Design review of the part built by this model. Coordinates are the model's own, in mm. A direction names the side the tool comes from. Coordinates: 2 decimals unless noted, no trailing zeros. Loops run counter-clockwise (first coordinate to the right, second up) from the corner with the lowest first, then second, coordinate; pieces in that order, holes last. Notation, with made-up numbers: M -30,48.5 L 9,48.5 A25 cw 9,79.5 Z; hole C -12,13.5 d5. An arc over 180 degrees is marked long. Put each result on its own line as item: value. Start each with the question number.
(1) Take a section at D-D, the plane z = -21. Give the boundary of the cut face in (x, y).
(2) Take a section at C-C, the plane x = -104. Give the boundary of the cut face in (y, z), then the cut area to 3 significant figures.
(3) Take a section at A-A, the plane y = 34.5. Give the boundary of the cut face in (x, z), then the cut area to 3 significant figures.
(4) Clearance check with flat-ended pins moving along their axes: pin 1 (4.5 mm diameter, centred on x = -11, z = 28.35, fed in from +Y); pin 2 (5.5 mm diameter, centred on y = 54.15, z = -25.11, fed in from +X); pin 3 (5 mm diameter, centred on x = -126, y = 72.5, fed in from -Z); pin 4 (2 mm diameter, centred on x = -129, z = -28.35, fed in from +Y). State where each tip first meets the part, or that it passes through.
(5) Take a section at B-B, the plane y = 66.5. Give the boundary of the cut face in (x, z).
(6) For faces 1 (the cylindrical face through (-17.787, 53.146, 26.424)), 2 (the flat face through (-69, 15, 0)), 3 (the flat face through (2, 2, 0)), 4 (the flat face through (-69, 17, 0)), list the 3-axis set-ups (+Z, -Z, +X, -X, +Y, -Y) from which the entire face can be reached by the end or side of a thin tool; tool diameter is ignored.
(7) The part is to be moulded in two halves that separate along Z. For faces 5 (the flat face through (-70, 16, -33.35)), 6 (the cylindrical face through (-10, 0.82, -29.66)), 7 (the flat face through (-20, 7, 0)), say which applies: +Z half, -Z half, draft (parallel to the pull), parting line (faces both ways), or undercut.
(8) For probe 1 along Z at (x, y) = (-155, 0.9); probe 2 along X at (y, z) = (13.5, -26); probe 3 along Y at (x, z) = (-122.5, 0), list the stretches that pass through material, from the lowest coordinate up. Write a range as [from, to].
```python
from build123d import *

# Parameters (mm, degrees)
SKETCH_1_W                   = 40
SKETCH_1_H                   = 66.7
EXTRUDE_1_DEPTH              = 2
SKETCH_2_W                   = 4
SKETCH_2_H                   = 66.7
EXTRUDE_2_DEPTH              = 100
CUT_EXTRUDE_1_DEPTH          = 115.526077816
CUT_EXTRUDE_1_DEPTH_BACK     = 115.526077816
HOLE_WIZARD_M4_1_D           = 3.3
HOLE_WIZARD_M4_1_CSINK_D     = 4.05
HOLE_WIZARD_M4_1_CSINK_ANGLE = 90
HOLE_WIZARD_M4_2_AT_2_COUNT  = 2
HOLE_WIZARD_M4_2_AT_2_PITCH  = 68.59294731
HOLE_WIZARD_M4_2_AT_3_COUNT  = 2
HOLE_WIZARD_M4_2_AT_3_PITCH  = 26
HOLE_WIZARD_M4_2_AT_4_COUNT  = 2
HOLE_WIZARD_M4_2_AT_4_PITCH  = 62.376998966
HOLE_WIZARD_M4_2_AT_5_COUNT  = 2
HOLE_WIZARD_M4_2_AT_5_PITCH  = 56.7
SKETCH_11_W                  = 66.7
SKETCH_11_H                  = 2
EXTRUDE_3_DEPTH              = 100
SKETCH_13_W                  = 40
SKETCH_13_H                  = 66.7
EXTRUDE_4_DEPTH              = 2
SKETCH_14_W                  = 4
SKETCH_14_H                  = 66.7
EXTRUDE_5_DEPTH              = 100
CUT_EXTRUDE_2_DEPTH          = 180.589037806
CUT_EXTRUDE_2_DEPTH_BACK     = 180.589037806
HOLE_WIZARD_M4_3_AT_2_COUNT  = 2
HOLE_WIZARD_M4_3_AT_2_PITCH  = 26
HOLE_WIZARD_M4_3_AT_3_COUNT  = 2
HOLE_WIZARD_M4_3_AT_3_PITCH  = 62.376998966
HOLE_WIZARD_M4_3_AT_4_COUNT  = 2
HOLE_WIZARD_M4_3_AT_4_PITCH  = 56.7
CUT_EXTRUDE_3_REACH          = 181.589
SKETCH_18_R                  = 9.5
CUT_EXTRUDE_4_REACH          = 181.589
SKETCH_21_R                  = 11
CUT_EXTRUDE_5_REACH          = 181.589
SKETCH_22_R                  = 4.5
FILLET_1_R                   = 2


with BuildPart() as part:
    # Sketch 1 → Extrude 1 (new body)
    with BuildSketch(Plane(origin=(0, 0, 0), x_dir=(1, 0, 0), z_dir=(0, 1, 0))):
        Rectangle(SKETCH_1_W, SKETCH_1_H)
    extrude(amount=EXTRUDE_1_DEPTH)

    # Sketch 2 → Extrude 2 (add)
    with BuildSketch(Plane(origin=(0, 2, 0), x_dir=(1, 0, 0), z_dir=(0, 1, 0))):
        with Locations((-18, 0)):
            Rectangle(SKETCH_2_W, SKETCH_2_H)
    extrude(amount=EXTRUDE_2_DEPTH)

    # Sketch 5 → Cut-Extrude 1 (cut, two sides: drawn at the far end of the back side and taken through both)
    with BuildSketch(Plane.ZY.offset(20).offset(-CUT_EXTRUDE_1_DEPTH_BACK)):
        with BuildLine():
            ThreePointArc((0, 102), (23.582011153, 92.232011153), (33.35, 68.65))
            Line((33.35, 68.65), (33.35, 102))
            Line((33.35, 102), (0, 102))
        make_face()
        with BuildLine():
            ThreePointArc((-33.35, 68.65), (-23.582011153, 92.232011153), (0, 102))
            Line((0, 102), (-33.35, 102))
            Line((-33.35, 102), (-33.35, 68.65))
        make_face()
    extrude(amount=CUT_EXTRUDE_1_DEPTH + CUT_EXTRUDE_1_DEPTH_BACK, mode=Mode.SUBTRACT)

    # Hole Wizard M4 _1 (through all)
    with Locations(Plane.ZY.offset(20)):
        with Locations((0, 97.65), (25.11473671, 54.15), (-25.11473671, 54.15)):
            CounterSinkHole(HOLE_WIZARD_M4_1_D / 2, HOLE_WIZARD_M4_1_CSINK_D / 2, counter_sink_angle=HOLE_WIZARD_M4_1_CSINK_ANGLE)

    # Sketch 10 → Hole Wizard M4 _2 (revolve, cut)
    with BuildSketch(Plane(origin=(15, 2, -28.35), x_dir=(0, 0, 1), z_dir=(1, 0, 0))):
        Polygon((0, 0), (0, 2), (1.65, 2), (1.65, 0.375), (2.025, 0), align=None)
    hole_wizard_m4_2 = revolve(axis=Axis((15, 8.35, -28.35), (0, -1, 0)), mode=Mode.SUBTRACT)

    # Hole Wizard M4 _2 at 2: Hole Wizard M4 _2 ×2
    with Locations(*[Vector(-0.9508085645250022, 0, 0.3097790722852413) * (i * HOLE_WIZARD_M4_2_AT_2_PITCH) for i in range(1, HOLE_WIZARD_M4_2_AT_2_COUNT)]):
        add(hole_wizard_m4_2, mode=Mode.SUBTRACT)

    # Hole Wizard M4 _2 at 3: Hole Wizard M4 _2 ×2
    with Locations(*[(-i * HOLE_WIZARD_M4_2_AT_3_PITCH, 0, 0) for i in range(1, HOLE_WIZARD_M4_2_AT_3_COUNT)]):
        add(hole_wizard_m4_2, mode=Mode.SUBTRACT)

    # Hole Wizard M4 _2 at 4: Hole Wizard M4 _2 ×2
    with Locations(*[Vector(-0.4168203092647413, 0, 0.9089889052042635) * (i * HOLE_WIZARD_M4_2_AT_4_PITCH) for i in range(1, HOLE_WIZARD_M4_2_AT_4_COUNT)]):
        add(hole_wizard_m4_2, mode=Mode.SUBTRACT)

    # Hole Wizard M4 _2 at 5: Hole Wizard M4 _2 ×2
    with Locations(*[(0, 0, i * HOLE_WIZARD_M4_2_AT_5_PITCH) for i in range(1, HOLE_WIZARD_M4_2_AT_5_COUNT)]):
        add(hole_wizard_m4_2, mode=Mode.SUBTRACT)

    # Sketch 11 → Extrude 3 (add)
    with BuildSketch(Plane.ZY.offset(20)):
        with Locations((0, 16)):
            Rectangle(SKETCH_11_W, SKETCH_11_H)
    extrude(amount=EXTRUDE_3_DEPTH)



with BuildPart() as body_2:
    # Sketch 13 → Extrude 4 (new body)
    with BuildSketch(Plane(origin=(0, 0, 0), x_dir=(1, 0, 0), z_dir=(0, 1, 0))):
        with Locations((-140, 0)):
            Rectangle(SKETCH_13_W, SKETCH_13_H)
    extrude(amount=EXTRUDE_4_DEPTH)


with BuildPart() as part_1:
    add(part.part)

    add(body_2.part)  # Extrude 5 merges body 2
    # Sketch 14 → Extrude 5 (add)
    with BuildSketch(Plane(origin=(0, 2, 0), x_dir=(1, 0, 0), z_dir=(0, 1, 0))):
        with Locations((-122, 0)):
            Rectangle(SKETCH_14_W, SKETCH_14_H)
    extrude(amount=EXTRUDE_5_DEPTH)

    # Sketch 15 → Cut-Extrude 2 (cut, two sides: drawn at the far end of the back side and taken through both)
    with BuildSketch(Plane.ZY.offset(124).offset(-CUT_EXTRUDE_2_DEPTH_BACK)):
        with BuildLine():
            ThreePointArc((0, 102), (23.582011153, 92.232011153), (33.35, 68.65))
            Line((33.35, 68.65), (33.35, 102))
            Line((33.35, 102), (0, 102))
        make_face()
        with BuildLine():
            ThreePointArc((-33.35, 68.65), (-23.582011153, 92.232011153), (0, 102))
            Line((0, 102), (-33.35, 102))
            Line((-33.35, 102), (-33.35, 68.65))
        make_face()
    extrude(amount=CUT_EXTRUDE_2_DEPTH + CUT_EXTRUDE_2_DEPTH_BACK, mode=Mode.SUBTRACT)

    # Sketch 17 → Hole Wizard M4 _3 (revolve, cut)
    with BuildSketch(Plane(origin=(-129, 2, -28.35), x_dir=(0, 0, 1), z_dir=(1, 0, 0))):
        Polygon((0, 0), (0, 2), (1.65, 2), (1.65, 0.375), (2.025, 0), align=None)
    hole_wizard_m4_3 = revolve(axis=Axis((-129, 8.35, -28.35), (0, -1, 0)), mode=Mode.SUBTRACT)

    # Hole Wizard M4 _3 at 2: Hole Wizard M4 _3 ×2
    with Locations(*[(-i * HOLE_WIZARD_M4_3_AT_2_PITCH, 0, 0) for i in range(1, HOLE_WIZARD_M4_3_AT_2_COUNT)]):
        add(hole_wizard_m4_3, mode=Mode.SUBTRACT)

    # Hole Wizard M4 _3 at 3: Hole Wizard M4 _3 ×2
    with Locations(*[Vector(-0.41682030926474106, 0, 0.9089889052042636) * (i * HOLE_WIZARD_M4_3_AT_3_PITCH) for i in range(1, HOLE_WIZARD_M4_3_AT_3_COUNT)]):
        add(hole_wizard_m4_3, mode=Mode.SUBTRACT)

    # Hole Wizard M4 _3 at 4: Hole Wizard M4 _3 ×2
    with Locations(*[(0, 0, i * HOLE_WIZARD_M4_3_AT_4_PITCH) for i in range(1, HOLE_WIZARD_M4_3_AT_4_COUNT)]):
        add(hole_wizard_m4_3, mode=Mode.SUBTRACT)

    # Sketch 18 → Cut-Extrude 3 (cut, up to next)
    with BuildSketch(Plane.ZY.offset(124), mode=Mode.PRIVATE) as cut_extrude_3_sk1:
        with Locations((0, 68.65)):
            Circle(SKETCH_18_R)
    cut_extrude_3_tool1 = extrude(cut_extrude_3_sk1.sketch, amount=-CUT_EXTRUDE_3_REACH, mode=Mode.PRIVATE) & part_1.part
    add(cut_extrude_3_tool1.solids().sort_by_distance((-124, 68.65, 0))[0], mode=Mode.SUBTRACT)

    # Sketch 21 → Cut-Extrude 4 (cut, up to next)
    with BuildSketch(Plane(origin=(-16, 0, 0), x_dir=(0, 0, -1), z_dir=(1, 0, 0)), mode=Mode.PRIVATE) as cut_extrude_4_sk1:
        with Locations((0, 68.65)):
            Circle(SKETCH_21_R)
    cut_extrude_4_tool1 = extrude(cut_extrude_4_sk1.sketch, amount=-CUT_EXTRUDE_4_REACH, mode=Mode.PRIVATE) & part_1.part
    add(cut_extrude_4_tool1.solids().sort_by_distance((-16, 68.65, 0))[0], mode=Mode.SUBTRACT)

    # Sketch 22 → Cut-Extrude 5 (cut, up to next)
    with BuildSketch(Plane(origin=(-16, 0, 0), x_dir=(0, 0, -1), z_dir=(1, 0, 0)), mode=Mode.PRIVATE) as cut_extrude_5_sk1:
        with Locations((-16.670989023, 59.025)):
            Circle(SKETCH_22_R)
    cut_extrude_5_tool1 = extrude(cut_extrude_5_sk1.sketch, amount=-CUT_EXTRUDE_5_REACH, mode=Mode.PRIVATE) & part_1.part
    add(cut_extrude_5_tool1.solids().sort_by_distance((-16, 59.025, 16.670989))[0], mode=Mode.SUBTRACT)

    # Fillet 1
    fillet_1_edges = [part_1.edges().sort_by_distance(p)[0] for p in [
        (-160, 1, -33.35),
        (-160, 1, 33.35),
        (20, 1, 33.35),
        (20, 1, -33.35),
    ]]
    fillet(fillet_1_edges, radius=FILLET_1_R)


solid = part_1.part
```
Computed values:
1. outline: M -160,0 L -120,0 L -120,15 L -20,15 L -20,0 L 20,0 L 20,2 L -16,2 L -16,94.56 L -20,94.56 L -20,17 L -120,17 L -120,94.56 L -124,94.56 L -124,2 L -160,2 Z
2. outline: M 15,-33.35 L 17,-33.35 L 17,33.35 L 15,33.35 Z
2. area: 133 mm^2
3. outline: M -124,-33.35 L -120,-33.35 L -120,33.35 L -124,33.35 Z; M -20,-33.35 L -16,-33.35 L -16,33.35 L -20,33.35 Z
3. area: 534 mm^2
4. pin 1: stops at y = 2
4. pin 2: stops at x = -16
4. pin 3: stops at z = -33.27
4. pin 4: passes through
5. outline: M -124,-33.35 L -120,-33.35 L -120,-9.25 L -124,-9.25 Z; M -124,9.25 L -120,9.25 L -120,33.35 L -124,33.35 Z; M -20,-33.35 L -16,-33.35 L -16,-10.79 L -20,-10.79 Z; M -20,10.79 L -16,10.79 L -16,33.35 L -20,33.35 Z
6. face 1: +X
6. face 2: +Z, -Z, -Y
6. face 3: +Z, -Z, +X, +Y
6. face 4: +Z, -Z, +Y
7. face 5: -Z half
7. face 6: undercut
7. face 7: draft
8. probe 1: z = [-33.35, -30], [-26.7, 26.7], [30, 33.35]
8. probe 2: x = [-124, -120], [-20, -16]
8. probe 3: y = [0, 59.15], [78.15, 102]
